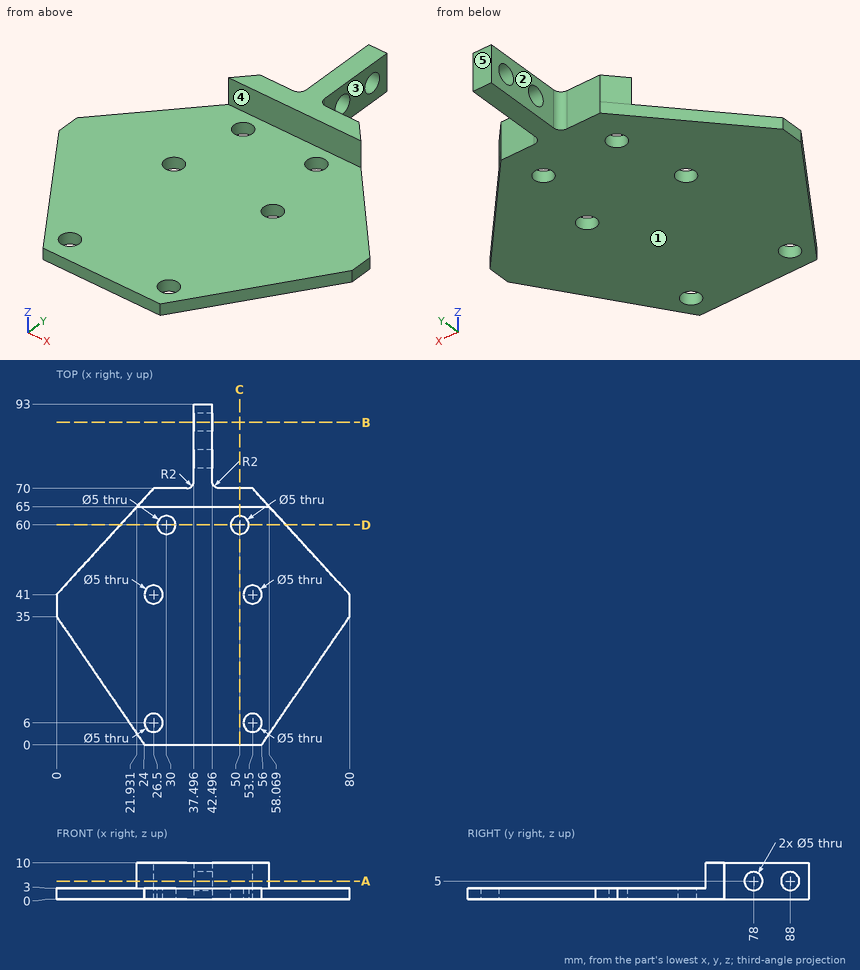
For this review, use the dimensioned drawing (mm, ordinates from the lowest corner) and the shaded views. A direction names the side the tool comes from. Give positions to 0.01 mm unless a question says otherwise; leave off trailing zeros. Loops run counter-clockwise (first coordinate to the right, second up) from the corner with the lowest first, then second, coordinate; pieces in that order, holes last. Notation, with made-up numbers: (4.5, 2) - (25.5, 2) arc R14 cw to (25.5, 20) - close; hole circle Ø7 at (42, -24.5). An arc over 180 degrees is marked (long way). Write each question's results on one line, items separated by ' | '.
(1) For line 1 along Y through (x, z) = (39.15, 5); line 2 along Y through (x, z) = (53.5, 0.7); line 3 along X through (y, z) = (5, 2), list the stretches that pass through material, from the lowest coordinate up.
Conclusion:
line 1: 65 to 75.5, 80.5 to 85.5, 90.5 to 93 | line 2: 0 to 3.5, 8.5 to 38.5, 43.5 to 70 | line 3: 20.57 to 24.21, 28.79 to 51.21, 55.79 to 59.43
(2) Take a section at D-D (y = 60). Give the boundary of the cut face in (x, z).
Conclusion:
outline: (17.36, 0) - (27.5, 0) - (27.5, 3) - (17.36, 3) - close; (32.5, 0) - (47.5, 0) - (47.5, 3) - (32.5, 3) - close; (52.5, 0) - (62.64, 0) - (62.64, 3) - (52.5, 3) - close
(3) Take a section at A-A (z = 5). Give the boundary of the cut face in (x, y) (1 decimal).
Conclusion:
outline: (21.9, 65) - (58.1, 65) - (53.5, 70) - (44.5, 70) arc R2 cw to (42.5, 72) - (42.5, 75.5) - (37.5, 75.5) - (37.5, 72) arc R2 cw to (35.5, 70) - (26.5, 70) - close; (37.5, 80.5) - (42.5, 80.5) - (42.5, 85.5) - (37.5, 85.5) - close; (37.5, 90.5) - (42.5, 90.5) - (42.5, 93) - (37.5, 93) - close
(4) For pin 1 Ø4.5 at (y, z) = (78, 5) entering from -X; pin 2 Ø2.5 at (x, z) = (50, 4.5) entering from +Y; pin 3 Ø5.5 at (x, z) = (32.5, 7) entering from -Y; pin 4 Ø6.5 at (x, y) = (53.5, 6) entering from +Z, all flat-tipped, find the tip position at first contact; note any pin that passes through.
Conclusion:
pin 1: through | pin 2: y = 70 | pin 3: y = 65 | pin 4: z = 3
(5) Take a section at B-B (y = 88). Give the boundary of the cut face in (x, z) (1 decimal).
Conclusion:
outline: (37.5, 0) - (42.5, 0) - (42.5, 2.5) - (37.5, 2.5) - close; (37.5, 7.5) - (42.5, 7.5) - (42.5, 10) - (37.5, 10) - close
(6) For the marked faces 1, 2, 3, 4 and 5, list the 3-axis set-ups (+Z, -Z, +X, -X, +Y, -Y) from which the entire face can be reached by the end or side of a thin tool; tool diameter is ignored.
Conclusion:
face 1: -Z, +X, -X, +Y, -Y | face 2: +Z, -Z, -X, +Y | face 3: +Z, -Z, +X, +Y | face 4: +Z, +X, -X, -Y | face 5: +Z, -Z, +X, -X, +Y
(7) Take a section at C-C (x = 50). Give the boundary of the cut face in (y, z).
Conclusion:
outline: (0, 0) - (57.5, 0) - (57.5, 3) - (0, 3) - close; (62.5, 0) - (70, 0) - (70, 10) - (65, 10) - (65, 3) - (62.5, 3) - close
